Work out the finished part from the listing and answer in its coordinate system (mm). Face numbers are marked on the shaded views. A direction names the side the tool comes from. Round coordinates to 2 decimals unless told otherwise and drop trailing zeros. Loops run counter-clockwise (first coordinate to the right, second up) from the corner with the lowest first, then second, coordinate; pieces in that order, holes last.
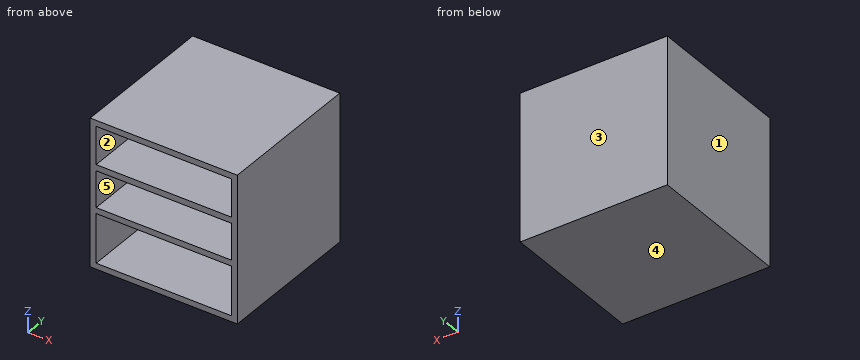
from build123d import *

# Parameters (mm, degrees)
F0_W     = 300
F0_H     = 300
F1_DEPTH = 300
F2_T     = -12
F3_W     = 276
F3_H     = 12.3312585362
F3_H_2   = 12
F4_DEPTH = 295


with BuildPart() as f1:
    # F0 (on Front) → F1 (new body)
    with BuildSketch(Plane.XZ):
        Rectangle(F0_W, F0_H)
    extrude(amount=-F1_DEPTH)

    # F2
    f2_openings = [f1.faces().sort_by_distance(p)[0] for p in [
        (0, 0, 0),
    ]]
    offset(amount=F2_T, openings=f2_openings)

    # F3 (on face) → F4 (join)
    with BuildSketch(Plane.XZ):
        with Locations((0, 54.6443801671)):
            Rectangle(F3_W, F3_H)
        with Locations((0, -31.8947338536)):
            Rectangle(F3_W, F3_H_2)
    extrude(amount=-F4_DEPTH)


solid = f1.part
Item 1: Section C-C, the plane x = -53 is taken. Give the vertices of the cut face in (y, z), plus the area to 3 significant figures.
Item 2: Section B-B, the plane z = 127 is taken. Give the vertices of the cut face in (x, y), plus the area to 3 significant figures.
Item 3: Section A-A, the plane y = 104.5 is taken. Give the vertices of the cut face in (x, z).
Item 4: Determine the mould class of the marked faces 1, 2 and 3 for opening direction X: pulls with the +X half, pulls with the -X half, needs draft (parallel to the pull), parting line crosses it, or undercut.
Item 5: For the marked faces 4 and 5, determine the directions among +Z, -Z, +X, -X, +Y, -Y from which every point of the face is accessible in a straight line to the end or side of a thin tool.
Item 6: Straight lines are drawn through the part: line 1 (Z direction, x = 118.5, y = 240); line 2 (X direction, y = 176, z = -78); line 3 (Y direction, x = 76.5, z = 67). For each, find the intervals that lie inside material, in ascending order.
Answer below:
1. outline: (0, -150) - (300, -150) - (300, 150) - (0, 150) - (0, 138) - (288, 138) - (288, 60.81) - (0, 60.81) - (0, 48.48) - (288, 48.48) - (288, -25.89) - (0, -25.89) - (0, -37.89) - (288, -37.89) - (288, -138) - (0, -138) - close
1. area: 17,500 mm2
2. outline: (-150, 0) - (-138, 0) - (-138, 288) - (138, 288) - (138, 0) - (150, 0) - (150, 300) - (-150, 300) - close
2. area: 10,500 mm2
3. outline: (-150, -150) - (150, -150) - (150, 150) - (-150, 150) - close; hole (-138, -138) - (138, -138) - (138, -37.89) - (-138, -37.89) - close; hole (-138, -25.89) - (138, -25.89) - (138, 48.48) - (-138, 48.48) - close; hole (-138, 60.81) - (138, 60.81) - (138, 138) - (-138, 138) - close
4. face 1: pulls with the -X half
4. face 2: undercut
4. face 3: needs draft
5. face 4: -Z, +X, -X, +Y, -Y
5. face 5: -Y
6. line 1: z = -150 to -138, -37.89 to -25.89, 48.48 to 60.81, 138 to 150
6. line 2: x = -150 to -138, 138 to 150
6. line 3: y = 288 to 300
